Here's how the part is built. I have some questions about the finished solid (model axes, mm). Face numbers are marked on the shaded views. A direction names the side the tool comes from. Coordinates: 2 decimals unless noted, no trailing zeros. Loops run counter-clockwise (first coordinate to the right, second up) from the corner with the lowest first, then second, coordinate; pieces in that order, holes last.
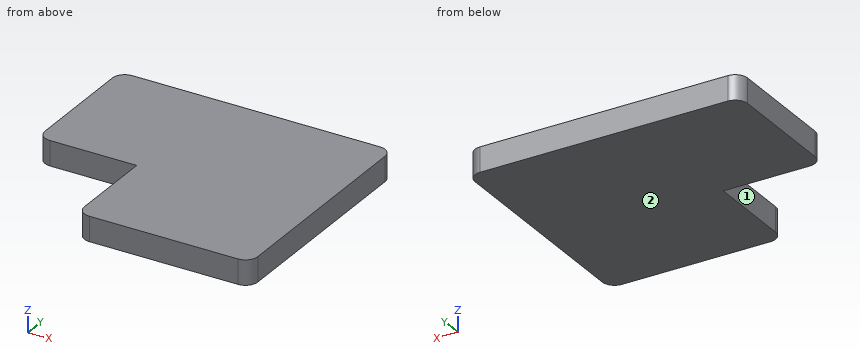
Autodesk Inventor part; units mm, degrees
ref_plane "YZ Plane" through (0, 0, 0) normal (1, 0, 0) x (0, 1, 0)
ref_plane "XZ Plane" through (0, 0, 0) normal (0, 1, 0) x (-1, 0, 0)
ref_plane "XY Plane" through (0, 0, 0) normal (0, 0, 1) x (1, 0, 0)
sketch "Schizzo1" plane through (0, 0, 0) normal (0, 0, 1) x (1, 0, 0)
  line L0 (0, 0) -> (-40, 0)
  line L1 (-40, 0) -> (-40, 55)
  line L2 (-40, 55) -> (70, 55)
  line L3 (70, 55) -> (70, -40)
  line L4 (70, -40) -> (0, -40)
  line L5 (0, -40) -> (0, 0)
  dimension "d0" = 40
  dimension "d1" = 40
  dimension "d2" = 55
  dimension "d3" = 70
extrude "Estrusione1" add sketch "Schizzo1" along normal blind 10
fillet "Raccordo1" radius 5 5 edges at (-40, 55, 5) (70, 55, 5) (70, -40, 5) (-40, 0, 5) (0, -40, 5)
properties part number "Supporto salita lama"
1. For pin 1 (5 mm diameter, centred on y = -6, z = 2, fed in from -X); pin 2 (12 mm diameter, centred on x = 42.5, y = -13.5, fed in from -Z); pin 3 (3 mm diameter, centred on x = -24.5, z = 3.5, fed in from -Y), each with a flat end and sliding along its axis, tell me the tip position at first contact or that it passes through.
2. I want a section at A-A (z = 5.5). Please give me the cut outline in (x, y).
3. I want a section at C-C (y = -29.5). Please give me the cut outline in (x, z).
4. On a 3-axis mill with a long thin cutter (end or side, diameter ignored), from which of +Z, -Z, +X, -X, +Y, -Y can I reach the whole of each face in a straight line? I mean the marked faces 1 and 2. Say none if no direction works.
5. I need wall thicknesses on line 1 along X through (y, z) = (-30.5, 3.75); line 2 along Y through (x, z) = (-30, 1.25). Which ranges of each line are inside material? Lowest first, please.
6. I want a section at B-B (x = -26). Please give me the cut outline in (y, z), then the cut area to 3 significant figures.
Response values:
1. pin 1: stops at x = 0
1. pin 2: stops at z = 0
1. pin 3: stops at y = 0
2. outline: (-40, 5) arc R5 ccw to (-35, 0) - (0, 0) - (0, -35) arc R5 ccw to (5, -40) - (65, -40) arc R5 ccw to (70, -35) - (70, 50) arc R5 ccw to (65, 55) - (-35, 55) arc R5 ccw to (-40, 50) - close
3. outline: (0, 0) - (70, 0) - (70, 10) - (0, 10) - close
4. face 1: +Z, -Z, -X, -Y
4. face 2: -Z, +X, -X, +Y, -Y
5. line 1: x = 0 to 70
5. line 2: y = 0 to 55
6. outline: (0, 0) - (55, 0) - (55, 10) - (0, 10) - close
6. area: 550 mm2
